For this review, take the finished solid that the model builds, in its own axes (mm). A direction names the side the tool comes from. Round coordinates to 2 decimals unless told otherwise and drop trailing zeros. Write each loop counter-clockwise with the first axis right and the second up, starting at its lowest first coordinate (ties: lowest second). Pieces come first, ordered by that corner, then holes. Notation, with made-up numbers: M -3.75,-10 L 22.25,-10 A31 cw 22.25,17 Z; hole C -10,81 d3. An arc over 180 degrees is marked long. Answer in a Markdown table with one row per item.
```python
from build123d import *

# Parameters (mm, degrees)
SKETCH1_R           = 12.5
BOSS_EXTRUDE1_DEPTH = 40
SKETCH2_R           = 19
CUT_EXTRUDE1_DEPTH  = 15
SKETCH3_W           = 5.2
SKETCH3_H           = 3.2
CUT_EXTRUDE2_DEPTH  = 7
SKETCH4_R           = 9.1
CUT_EXTRUDE3_DEPTH  = 15


with BuildPart() as part:
    # Sketch1 → Boss-Extrude1 (new body)
    with BuildSketch(Plane.XY):
        Circle(SKETCH1_R)
    extrude(amount=BOSS_EXTRUDE1_DEPTH)

    # Sketch2 → Cut-Extrude1 (cut)
    with BuildSketch(Plane.XY.offset(40)):
        Circle(SKETCH2_R)
    extrude(amount=-CUT_EXTRUDE1_DEPTH, mode=Mode.SUBTRACT)

    # Sketch3 → Cut-Extrude2 (cut)
    with BuildSketch(Plane(origin=(0, 0, 0), x_dir=(-1, 0, 0), z_dir=(0, 0, -1))):
        Rectangle(SKETCH3_W, SKETCH3_H)
    extrude(amount=-CUT_EXTRUDE2_DEPTH, mode=Mode.SUBTRACT)

    # Sketch4 → Cut-Extrude3 (cut)
    with BuildSketch(Plane.XY.offset(25)):
        Circle(SKETCH4_R)
    extrude(amount=-CUT_EXTRUDE3_DEPTH, mode=Mode.SUBTRACT)


solid = part.part
```
Q1. Take a section at B-B (x = 0). State the section outline as (y, z) points.
Found:
| item | result |
|---|---|
| outline | M -12.5,0 L -1.6,0 L -1.6,7 L 1.6,7 L 1.6,0 L 12.5,0 L 12.5,25 L 9.1,25 L 9.1,10 L -9.1,10 L -9.1,25 L -12.5,25 Z |
Q2. Take a section at D-D (z = 9.25). State the section outline as (x, y) points, then the cut area to 3 significant figures.
Found:
| item | result |
|---|---|
| outline | C 0,0 d25 |
| area | 491 mm² |
Q3. Take a section at A-A (y = 0). State the section outline as (x, z) points, then the cut area to 3 significant figures.
Found:
| item | result |
|---|---|
| outline | M -12.5,0 L -2.6,0 L -2.6,7 L 2.6,7 L 2.6,0 L 12.5,0 L 12.5,25 L 9.1,25 L 9.1,10 L -9.1,10 L -9.1,25 L -12.5,25 Z |
| area | 316 mm² |
Q4. Insertion check: P1, Ø2, axis at x = 4, y = 2, coming from the +Z side; P2, Ø12, axis at x = -7, z = 12, coming from the +Y side; P3, Ø1, axis at x = -5.5, z = 14.5, coming from the -Y side. Each pin has a flat end and moves straight along its axis. Give the tip position at first contact, or say it passes through.
Found:
| item | result |
|---|---|
| P1 | z = 10 |
| P2 | y = 12.46 |
| P3 | y = -11.46 |
Q5. Mouldability with a two-part tool opening along X and no side actions: class faces 1 (the face through (0, -1.6, 3)), 2 (the face through (0, -3, 0)), 3 (the face through (11.923, 3.755, 12.325)) as +X half, -X half, draft (parallel to the pull), parting line (faces both ways), or undercut.
Found:
| item | result |
|---|---|
| face 1 | undercut |
| face 2 | draft |
| face 3 | parting line |
Q6. For probe 1 along Y at (x, z) = (0, 21.75); probe 2 along Z at (x, y) = (8.5, -2); probe 3 along X at (y, z) = (8, 19.5), list the stretches that pass through material, from the lowest coordinate up.
Found:
| item | result |
|---|---|
| probe 1 | -12.5 to -9.1, 9.1 to 12.5 |
| probe 2 | 0 to 10 |
| probe 3 | -9.6 to -4.34, 4.34 to 9.6 |
Q7. Machinability: for faces 4 (the face through (-1.973, -8.884, 17.605)), 5 (the face through (-1.9, -9.2, 25)), 6 (the face through (-2.6, 0, 3)), which of the approach directions +Z, -Z, +X, -X, +Y, -Y give a long, thin tool a straight path to every point of the face, cutting with its end or side? Answer none if there is none.
Found:
| item | result |
|---|---|
| face 4 | +Z |
| face 5 | +Z, +X, -X, +Y, -Y |
| face 6 | -Z |
Q8. Take a section at C-C (z = 22.5). State the section outline as (x, y) points.
Found:
| item | result |
|---|---|
| outline | C 0,0 d25; hole C 0,0 d18.2 |
